Job drawing, mm, ordinate dimensions from the low corner. One solid piece. Give positions to 0.01 mm unless a question says otherwise; leave off trailing zeros. Write each loop counter-clockwise with the first axis right and the second up, starting at its lowest first coordinate (ties: lowest second). Pieces come first, ordered by that corner, then holes. Notation, with made-up numbers: (84, 0) -> (124, 0) arc R15 ccw to (124, 8) -> close; hole circle Ø11 at (26, -17). An arc over 180 degrees is marked (long way). Put each result on its own line as item: value. Start each with the question number.
Item 1: Flat gauge pins, fed straight in: pin 1 Ø3 at (y, z) = (5, 2) entering from -X; pin 2 Ø2 at (y, z) = (4.318, 2.54) entering from +X. Where does each tip first touch, or does it go through?
Item 2: Slice it at A-A, the plane y = 6.75. List the corners of the cut face in (x, z), plus the area to 3 significant figures.
Item 3: Drill centre lines: line 1 along X through (y, z) = (3.75, 4.35); line 2 along Z through (x, y) = (2.9, 4.25); line 3 along Y through (x, z) = (2.1, 3.15). Where is each one in solid material? Low to high.
Item 4: Two-plate mould, pull along Z, no slides. Class the marked faces 1, 2 and 3: pulls with the +Z half, pulls with the -Z half, needs draft (parallel to the pull), parting line crosses it, or undercut.
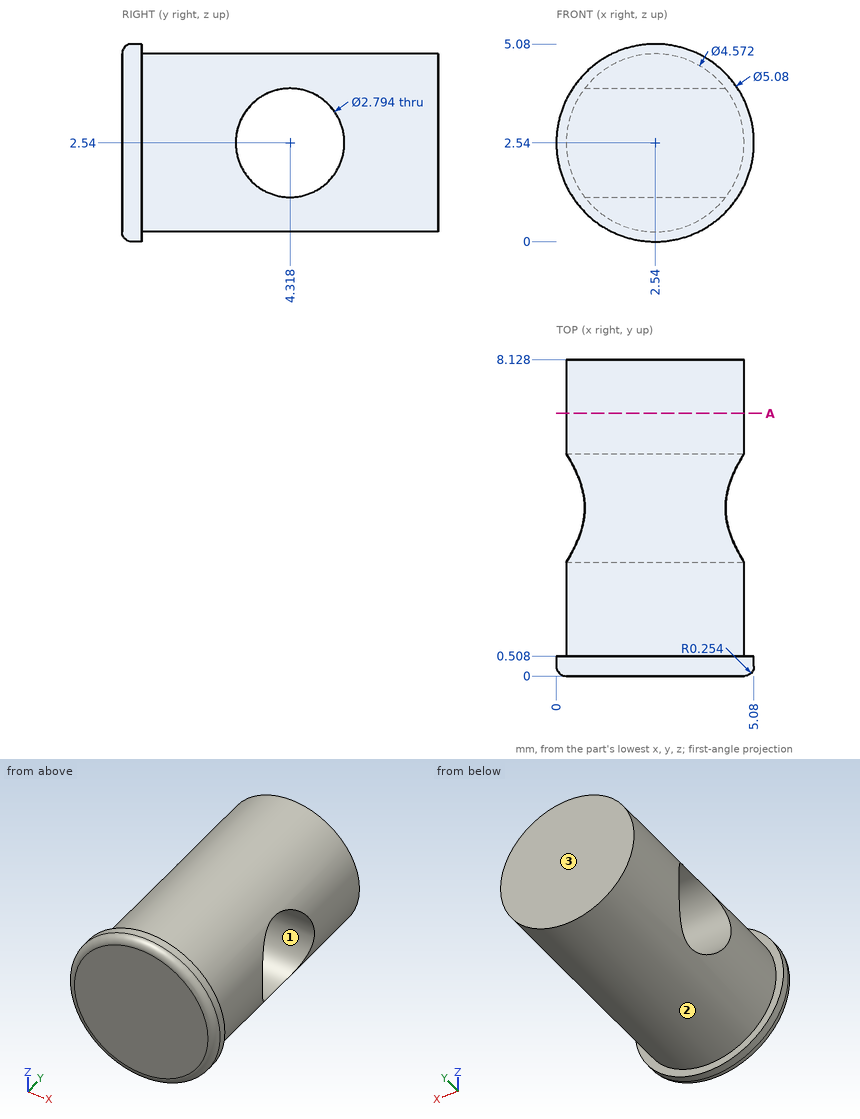
Values follow:
1. pin 1: x = 0.25
1. pin 2: through
2. outline: circle Ø4.57 at (2.54, 2.54)
2. area: 16.4 mm2
3. line 1: 1.14 to 3.94
3. line 2: 0.28 to 1.14, 3.94 to 4.8
3. line 3: 0 to 3.06, 5.57 to 8.13
4. face 1: undercut
4. face 2: parting line crosses it
4. face 3: needs draft
